from build123d import *

# Parameters (mm, degrees)
CYLINDER054061_R                           = 1.3
CYLINDER054061_DEPTH                       = 50
CYLINDER054060_R                           = 2.2
CYLINDER054060_DEPTH                       = 20
CYLINDER054060_PITCH_ANGLE                 = 90
CYLINDER054056_R                           = 1.4
CYLINDER054056_DEPTH                       = 40
CYLINDER054056_PITCH_ANGLE                 = 90
BOX112015002017004007004036_W              = 60
BOX112015002017004007004036_H              = 14
BOX112015002017004007004036_DEPTH          = 8
BOX112015002017004007004036_PITCH_ANGLE    = 90
BOX112015002017004007004037_W              = 10
BOX112015002017004007004037_H              = 28
BOX112015002017004007004037_DEPTH          = 16
BOX112015002017004007004037_PITCH_ANGLE    = 90
CHAMFER006012025_SIZE                      = 8
CHAMFER006012026_SIZE                      = 8
CONE012_PITCH_ANGLE                        = 90
PART_MIRRORING005008_PITCH_ANGLE           = 90
BOX112015002017004007004038008_W           = 10
BOX112015002017004007004038008_H           = 28
BOX112015002017004007004038008_DEPTH       = 16
BOX112015002017004007004038008_PITCH_ANGLE = 90


with BuildPart() as cylinder054101:
    # Cylinder054061 → Cylinder054061 (new body)
    with BuildSketch(Plane(origin=(0, -10.5, 7), x_dir=(1, 0, 0), z_dir=(0, 0, 1))):
        Circle(CYLINDER054061_R)
    extrude(amount=CYLINDER054061_DEPTH)


with BuildPart() as cylinder054100:
    # Cylinder054060 → Cylinder054060 (new body)
    with BuildSketch(Plane.XY):
        Circle(CYLINDER054060_R)
    extrude(amount=CYLINDER054060_DEPTH)


with BuildPart() as cylinder054100_1:
    # Cylinder054060 pitch: moved
    add(cylinder054100.part.rotate(Axis((0, 0, 0), (0, 1, 0)), CYLINDER054060_PITCH_ANGLE))


with BuildPart() as cylinder054100_2:
    # Cylinder054060 placement: moved
    add(cylinder054100_1.part.moved(Location((-10, 11, 32))))


with BuildPart() as bearing_m3:
    # Cylinder054056 → Cylinder054056 (new body)
    with BuildSketch(Plane.XY):
        Circle(CYLINDER054056_R)
    extrude(amount=CYLINDER054056_DEPTH)


with BuildPart() as bearing_m3_1:
    # Cylinder054056 pitch: moved
    add(bearing_m3.part.rotate(Axis((0, 0, 0), (0, 1, 0)), CYLINDER054056_PITCH_ANGLE))


with BuildPart() as bearing_m3_2:
    # Cylinder054056 placement: moved
    add(bearing_m3_1.part.moved(Location((-20, 0, 38))))


with BuildPart() as cube119:
    # Box112015002017004007004036 → Box112015002017004007004036 (new body)
    with BuildSketch(Plane.XY):
        with Locations((30, 7)):
            Rectangle(BOX112015002017004007004036_W, BOX112015002017004007004036_H)
    extrude(amount=BOX112015002017004007004036_DEPTH)


with BuildPart() as cube119_1:
    # Box112015002017004007004036 pitch: moved
    add(cube119.part.rotate(Axis((0, 0, 0), (0, 1, 0)), BOX112015002017004007004036_PITCH_ANGLE))


with BuildPart() as cube119_2:
    # Box112015002017004007004036 placement: moved
    add(cube119_1.part.moved(Location((-4, -7, 68))))


with BuildPart() as cut298:
    # Box112015002017004007004037 → Box112015002017004007004037 (new body)
    with BuildSketch(Plane.XY):
        with Locations((5, 14)):
            Rectangle(BOX112015002017004007004037_W, BOX112015002017004007004037_H)
    extrude(amount=BOX112015002017004007004037_DEPTH)


with BuildPart() as cut298_1:
    # Box112015002017004007004037 pitch: moved
    add(cut298.part.rotate(Axis((0, 0, 0), (0, 1, 0)), BOX112015002017004007004037_PITCH_ANGLE))


with BuildPart() as cut298_2:
    # Box112015002017004007004037 placement: moved
    add(cut298_1.part.moved(Location((-8, -14, 43))))

    # Chamfer006012025
    chamfer006012025_edges = [cut298_2.edges().sort_by_distance(p)[0] for p in [
        (8, 14, 38),
    ]]
    chamfer(chamfer006012025_edges, length=CHAMFER006012025_SIZE)

    # Chamfer006012026
    chamfer006012026_edges = [cut298_2.edges().sort_by_distance(p)[0] for p in [
        (8, -14, 38),
    ]]
    chamfer(chamfer006012026_edges, length=CHAMFER006012026_SIZE)

    # Cut298: cut Cube119
    add(cube119_2.part, mode=Mode.SUBTRACT)


with BuildPart() as cone012:
    # Cone012 → Cone012 (revolve)
    with BuildSketch(Plane.XZ):
        Polygon((0, 0), (2.5, 0), (5.5, 3), (0, 3), align=None)
    revolve(axis=Axis((0, 0, 0), (0, 0, 1)))


with BuildPart() as cone012_1:
    # Cone012 pitch: moved
    add(cone012.part.rotate(Axis((0, 0, 0), (0, 1, 0)), CONE012_PITCH_ANGLE))


with BuildPart() as cone012_2:
    # Cone012 placement: moved
    add(cone012_1.part.moved(Location((1.9, 0, 38))))


with BuildPart() as cone011:
    # Cone011 → Cone011 (revolve)
    with BuildSketch(Plane(origin=(0, 0, 2), x_dir=(1, 0, 0), z_dir=(0, -1, 0))):
        Polygon((0, 0), (2.5, 0), (5.5, 3), (0, 3), align=None)
    revolve(axis=Axis((0, 0, 2), (0, 0, 1)))


with BuildPart() as bearing_cones:
    # Part__Mirroring005008: instance of Cone011
    add(cone011.part.mirror(Plane(origin=(0, 0, 0), x_dir=(0, 1, 0), z_dir=(0, 0, 1))))


with BuildPart() as bearing_cones_1:
    # Part__Mirroring005008 pitch: moved
    add(bearing_cones.part.rotate(Axis((0, 0, 0), (0, 1, 0)), PART_MIRRORING005008_PITCH_ANGLE))


with BuildPart() as bearing_cones_2:
    # Part__Mirroring005008 placement: moved
    add(bearing_cones_1.part.moved(Location((0.1, 0, 38))))

    # Fusion051010010012015014027: union Cone012
    add(cone012_2.part)


with BuildPart() as f_6144_wire_tensioner_block:
    # Box112015002017004007004038008 → Box112015002017004007004038008 (new body)
    with BuildSketch(Plane.XY):
        with Locations((5, 14)):
            Rectangle(BOX112015002017004007004038008_W, BOX112015002017004007004038008_H)
    extrude(amount=BOX112015002017004007004038008_DEPTH)


with BuildPart() as f_6144_wire_tensioner_block_1:
    # Box112015002017004007004038008 pitch: moved
    add(f_6144_wire_tensioner_block.part.rotate(Axis((0, 0, 0), (0, 1, 0)), BOX112015002017004007004038008_PITCH_ANGLE))


with BuildPart() as f_6144_wire_tensioner_block_2:
    # Box112015002017004007004038008 placement: moved
    add(f_6144_wire_tensioner_block_1.part.moved(Location((-8, -14, 43))))

    # Common010: intersect bearing-cones
    add(bearing_cones_2.part, mode=Mode.INTERSECT)

    # Fusion051010010012015014034: union Cut298
    add(cut298_2.part)

    # Cut299: cut bearing-M3
    add(bearing_m3_2.part, mode=Mode.SUBTRACT)

    # Cut300: cut Cylinder054100
    add(cylinder054100_2.part, mode=Mode.SUBTRACT)

    # Cut301: cut Cylinder054101
    add(cylinder054101.part, mode=Mode.SUBTRACT)


with BuildPart() as f_6144_wire_tensioner_block_3:
    # Cut301 placement: moved
    add(f_6144_wire_tensioner_block_2.part.moved(Location((0, 0, 79))))


solid = f_6144_wire_tensioner_block_3.part
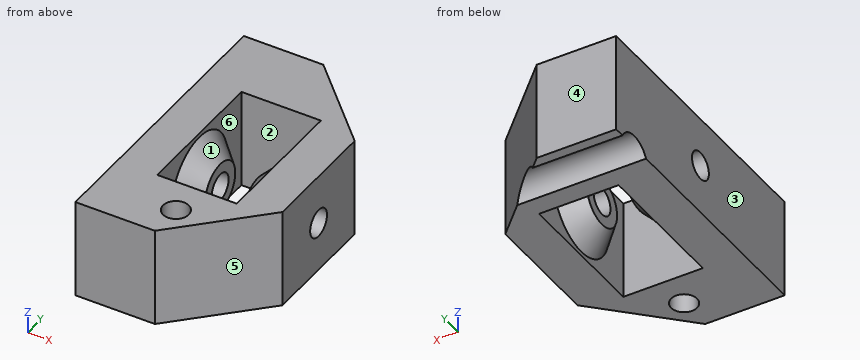
Geometry check sheet. Reference: the model listing, model coordinates, mm. Face numbers are marked on the shaded views. A direction names the side the tool comes from. Give positions to 0.01 mm unless a question says otherwise; leave off trailing zeros. Loops run counter-clockwise (first coordinate to the right, second up) from the corner with the lowest first, then second, coordinate; pieces in that order, holes last. Notation, with made-up numbers: M 35,63.5 L 62,63.5 A24 cw 62,80.5 Z; hole C 66.5,25.25 d3. An arc over 180 degrees is marked long. Answer as a JSON object with one key per item and string values. Group by question number.
Item 1: Sectioned sample at D-D on y = 0. Record the boundary of the cut face in (x, z), plus the area to 3 significant figures.
Item 2: Material ranges on L1, parallel to X at y = 4.5, z = 118.25; L2, parallel to Z at x = -6.25, y = 0; L3, parallel to Y at x = -5.5, z = 117, recorded low to high.
Item 3: Sectioned sample at A-A on x = -2.75. Record the boundary of the cut face in (y, z).
Item 4: Gauge pin test, flat end, axial feed: pin 1 (3 mm diameter, centred on x = 2, z = 114.5, fed in from -Y). Record the tip position at first contact, or that the pin passes through.
Item 5: Sectioned sample at B-B on z = 117. Record the boundary of the cut face in (x, y), plus the area to 3 significant figures.
Item 6: Access from +Z, -Z, +X, -X, +Y, -Y to the whole of each face (thin tool, end or side, straight path). Record for the marked faces 1, 2 and 3.
Item 7: Sectioned sample at C-C on x = -0.5. Record the boundary of the cut face in (y, z), plus the area to 3 significant figures.
Item 8: Mould release check, pull along X, two halves, no side actions. Record for the marked faces 4, 5 and 6: pulls with the +X half, pulls with the -X half, needs draft (parallel to the pull), parting line crosses it, or undercut.
Findings below:
{
 "1": {"outline": "M -8,112 L -4,112 L -4,112.4 L -1.9,114.5 L -1.9,115.6 L -8,115.6 Z; M -8,118.4 L -1.9,118.4 L -1.9,119.5 L -4,121.6 L -4,122 L -8,122 Z; M 1.9,114.5 L 4,112.4 L 4,112 L 8,112 L 8,115.6 L 1.9,115.6 Z; M 1.9,118.4 L 8,118.4 L 8,122 L 4,122 L 4,121.6 L 1.9,119.5 Z", "area": "75.7 mm2"},
 "2": {"L1": "-8 to -4, 4 to 8", "L2": "112 to 115.6, 118.4 to 122", "L3": "-14 to -1.4, 1.4 to 14"},
 "3": {"outline": "M -14,112 L -7,112 L -7,122 L -14,122 Z; C 0,117 d6.7; M 7,112 L 9.04,112 A2.2 cw 12.96,112 L 14,112 L 14,122 L 7,122 Z; hole C 0,117 d2.8"},
 "4": {"pin 1": "y = -13.5"},
 "5": {"outline": "M -8,-14 L 0,-14 L 8,-6 L 8,-1.4 L 1.9,-1.4 L 1.9,-2.5 L 4,-4.6 L 4,-7 L -4,-7 L -4,-4.6 L -1.9,-2.5 L -1.9,-1.4 L -8,-1.4 Z; M -8,1.4 L -1.9,1.4 L -1.9,2.5 L -4,4.6 L -4,7 L 4,7 L 4,4.6 L 1.9,2.5 L 1.9,1.4 L 8,1.4 L 8,6 L 0,14 L -8,14 Z; hole C 0,-10.5 d2.6", "area": "262 mm2"},
 "6": {"face 1": "none", "face 2": "+Z, -Z", "face 3": "+Z, -Z, -X, +Y, -Y"},
 "7": {"outline": "M -14,112 L -11.7,112 L -11.7,122 L -14,122 Z; M -9.3,112 L -7,112 L -7,122 L -9.3,122 Z; M 7,112 L 9.04,112 A2.2 cw 12.96,112 L 14,112 L 14,122 L 7,122 Z", "area": "113 mm2"},
 "8": {"face 4": "needs draft", "face 5": "pulls with the +X half", "face 6": "undercut"}
}
